Could you check a few things on this drawing? It's one solid part, dimensions in mm from its lowest x, y, z. Coordinates: 2 decimals unless noted, no trailing zeros. Order: outer loops, then holes, each group sorted by start corner. A loop starts at its lowest first (then second) coordinate and runs counter-clockwise, first axis right, second up. Notation, with made-up numbers: (-32, 36) - (27, 36) arc R10 cw to (27, 44) - close; hole circle Ø6 at (85, 60.5). An arc over 180 degrees is marked (long way). Answer in a Markdown table with one row per item. Add a question column.
Item 1: I want a section at B-B (z = 2.5). Please give me the cut outline in (x, y) (3 decimals).
Item 2: Will these pins go through, and if not, where does the flat tip stop? pin 1 Ø10 at (x, y) = (65, 18.5) entering from -Z; pin 2 Ø7.5 at (x, y) = (72, 18.5) entering from +Z; pin 3 Ø10 at (x, y) = (88.5, 19) entering from -Z; pin 4 Ø1.5 at (y, z) = (9, 3) entering from -X.
Item 3: I want a section at C-C (y = 9). Please give me the cut outline in (x, z), plus the area to 3 significant figures.
Item 4: I want a section at D-D (x = 64). Please give me the cut outline in (y, z) (3 decimals).
Item 5: If I drill on line 1 along X through (y, z) = (21, 3.95); line 2 along Y through (x, z) = (73, 2.9) (3 decimals); line 3 along X through (y, z) = (9.5, 3.05), over which ranges is the centre line in solid material (lowest first)? Write a range as from..to.
Item 6: Thinking about a two-plate mould opening in Z: for the marked faces 1, 2 and 3, which applies, +Z half, -Z half, draft (parallel to the pull), parting line (faces both ways), or undercut?
Item 7: I want a section at A-A (y = 19). Please give me the cut outline in (x, z), plus the area to 3 significant figures.
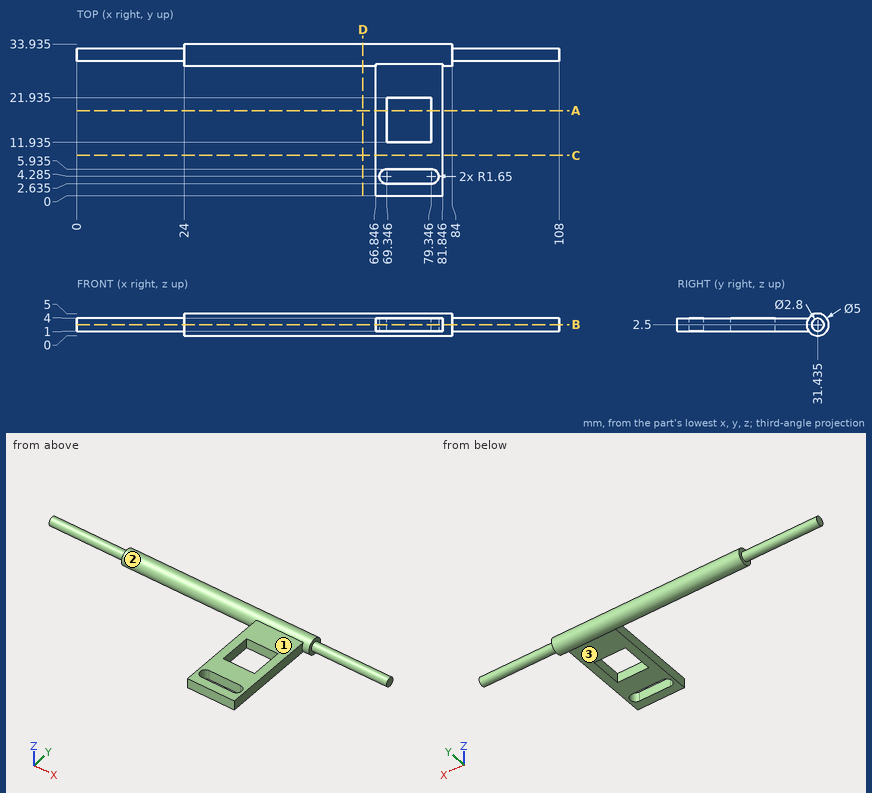
Values follow:
| question | item | result |
|---|---|---|
| 1 | outline | (0, 30.035) - (24, 30.035) - (24, 28.935) - (66.846, 28.935) - (66.846, 0) - (81.846, 0) - (81.846, 28.935) - (84, 28.935) - (84, 30.035) - (108, 30.035) - (108, 32.835) - (84, 32.835) - (84, 33.935) - (24, 33.935) - (24, 32.835) - (0, 32.835) - close; hole (69.346, 2.635) - (79.346, 2.635) arc R1.65 ccw to (79.346, 5.935) - (69.346, 5.935) arc R1.65 ccw to start; hole (69.346, 11.935) - (79.346, 11.935) - (79.346, 21.935) - (69.346, 21.935) - close |
| 2 | pin 1 | stops at z = 1 |
| 2 | pin 2 | stops at z = 4 |
| 2 | pin 3 | passes through |
| 2 | pin 4 | stops at x = 66.85 |
| 3 | outline | (66.85, 1) - (81.85, 1) - (81.85, 4) - (66.85, 4) - close |
| 3 | area | 45.0 mm^2 |
| 4 | outline | circle Ø5 at (31.435, 2.5) |
| 5 | line 1 | x = 66.85..69.35, 79.35..81.85 |
| 5 | line 2 | y = 0..2.635, 5.935..11.935, 21.935..33.903 |
| 5 | line 3 | x = 66.85..81.85 |
| 6 | face 1 | +Z half |
| 6 | face 2 | parting line |
| 6 | face 3 | -Z half |
| 7 | outline | (66.85, 1) - (69.35, 1) - (69.35, 4) - (66.85, 4) - close; (79.35, 1) - (81.85, 1) - (81.85, 4) - (79.35, 4) - close |
| 7 | area | 15.0 mm^2 |
